from build123d import *

# Parameters (mm, degrees)
SKETCH1_W           = 288
SKETCH1_H           = 50
BOSS_EXTRUDE1_DEPTH = 5
SKETCH2_R           = 1.5
CUT_EXTRUDE1_DEPTH  = 5
SKETCH3_W           = 30
SKETCH3_H           = 45
BOSS_EXTRUDE2_DEPTH = 5
FILLET1_R           = 10
SKETCH4_W           = 5
SKETCH4_H           = 5
CUT_EXTRUDE2_DEPTH  = 5
SKETCH5_R           = 1.7
CUT_EXTRUDE3_DEPTH  = 5
SKETCH7_R           = 2
CUT_EXTRUDE4_DEPTH  = 10


with BuildPart() as part:
    # Sketch1 → Boss-Extrude1 (new body)
    with BuildSketch(Plane(origin=(0, 0, 0), x_dir=(1, 0, 0), z_dir=(0, 1, 0))):
        Rectangle(SKETCH1_W, SKETCH1_H)
    extrude(amount=BOSS_EXTRUDE1_DEPTH)

    # Sketch2 → Cut-Extrude1 (cut)
    with BuildSketch(Plane(origin=(0, 5, 0), x_dir=(1, 0, 0), z_dir=(0, 1, 0))):
        with Locations((-130, 10)):
            Circle(SKETCH2_R)
        with Locations((-110, 10)):
            Circle(SKETCH2_R)
        with Locations((-110, -10)):
            Circle(SKETCH2_R)
        with Locations((-130, -10)):
            Circle(SKETCH2_R)
        with Locations((130, -10)):
            Circle(SKETCH2_R)
        with Locations((110, -10)):
            Circle(SKETCH2_R)
        with Locations((110, 10)):
            Circle(SKETCH2_R)
        with Locations((130, 10)):
            Circle(SKETCH2_R)
    extrude(amount=-CUT_EXTRUDE1_DEPTH, mode=Mode.SUBTRACT)

    # Sketch3 → Boss-Extrude2 (add)
    with BuildSketch(Plane(origin=(0, 5, 0), x_dir=(1, 0, 0), z_dir=(0, 1, 0))):
        with Locations((-129, 47.5)):
            Rectangle(SKETCH3_W, SKETCH3_H)
        with Locations((-129, -47.5)):
            Rectangle(SKETCH3_W, SKETCH3_H)
        with Locations((129, -47.5)):
            Rectangle(SKETCH3_W, SKETCH3_H)
        with Locations((129, 47.5)):
            Rectangle(SKETCH3_W, SKETCH3_H)
    extrude(amount=-BOSS_EXTRUDE2_DEPTH)

    # Fillet1
    fillet1_edges = [part.edges().sort_by_distance(p)[0] for p in [
        (-114, 2.5, -25),
        (-114, 2.5, 25),
        (114, 2.5, 25),
        (114, 2.5, -25),
    ]]
    fillet(fillet1_edges, radius=FILLET1_R)

    # Sketch4 → Cut-Extrude2 (cut)
    with BuildSketch(Plane(origin=(0, 5, 0), x_dir=(1, 0, 0), z_dir=(0, 1, 0))):
        with Locations((10, 10)):
            Rectangle(SKETCH4_W, SKETCH4_H)
        with Locations((-10, 10)):
            Rectangle(SKETCH4_W, SKETCH4_H)
        with Locations((-10, -10)):
            Rectangle(SKETCH4_W, SKETCH4_H)
        with Locations((10, -10)):
            Rectangle(SKETCH4_W, SKETCH4_H)
    extrude(amount=-CUT_EXTRUDE2_DEPTH, mode=Mode.SUBTRACT)

    # Sketch5 → Cut-Extrude3 (cut)
    with BuildSketch(Plane(origin=(0, 5, 0), x_dir=(1, 0, 0), z_dir=(0, 1, 0))):
        with Locations((0, 10)):
            Circle(SKETCH5_R)
        with Locations((0, -10)):
            Circle(SKETCH5_R)
        with Locations((10, 0)):
            Circle(SKETCH5_R)
        with Locations((-10, 0)):
            Circle(SKETCH5_R)
    extrude(amount=-CUT_EXTRUDE3_DEPTH, mode=Mode.SUBTRACT)

    # Sketch7 → Cut-Extrude4 (cut)
    with BuildSketch(Plane(origin=(0, 5, 0), x_dir=(1, 0, 0), z_dir=(0, 1, 0))):
        with Locations((-136.5, 45)):
            Circle(SKETCH7_R)
        with Locations((-136.5, -30)):
            Circle(SKETCH7_R)
        with Locations((136.5, -30)):
            Circle(SKETCH7_R)
        with Locations((136.5, 45)):
            Circle(SKETCH7_R)
    extrude(amount=-CUT_EXTRUDE4_DEPTH, mode=Mode.SUBTRACT)


solid = part.part
Geometry: final body of the model. Coordinates: model frame, mm. A direction names the side the tool comes from. Give positions to 0.01 mm unless a question says otherwise; leave off trailing zeros. Loops run counter-clockwise (first coordinate to the right, second up) from the corner with the lowest first, then second, coordinate; pieces in that order, holes last. Notation, with made-up numbers: M 16.25,62.5 L 74.25,62.5 A27 cw 74.25,89.5 Z; hole C 69,50.25 d3. An arc over 180 degrees is marked long. Put each result on its own line as item: value.
1) Cut plane C-C, the plane x = 73. Return the cut outline in (y, z), plus the area to 3 significant figures.
Computed values:
outline: M 0,-25 L 5,-25 L 5,25 L 0,25 Z
area: 250 mm^2
2) Cut plane B-B, the plane y = 4.1. Give the number of separate pieces and of enclosed holes in the cut face, plus the area to 3 significant figures.
Computed values:
separate pieces: 1
enclosed holes: 20
area: 19,600 mm^2
3) Mould query, pull axis X, two halves, no side actions, for faces 5 (the flat face through (10, 3, 12.5)), 6 (the flat face through (-10, 3, 7.5)), 7 (the flat face through (-144, 3, 1)), 8 (the flat face through (129, 3, -70)). Classes: released by +X, released by -X, zero draft, split by the parting line, or undercut.
Computed values:
face 5: undercut
face 6: undercut
face 7: released by -X
face 8: zero draft
4) Cut plane A-A, the plane z = 58. Return the cut outline in (x, y), plus the area to 3 significant figures.
Computed values:
outline: M -144,0 L -114,0 L -114,5 L -144,5 Z; M 114,0 L 144,0 L 144,5 L 114,5 Z
area: 300 mm^2
5) Material intervals for L1, parallel to Z at x = -136.5, y = 2.85; L2, parallel to Z at x = 0, y = 2.45; L3, parallel to Z at x = 10, y = 1.6, sorted ascending. Write a range as from..to.
Computed values:
L1: z = -70..-47, -43..28, 32..70
L2: z = -25..-11.7, -8.3..8.3, 11.7..25
L3: z = -25..-12.5, -7.5..-1.7, 1.7..7.5, 12.5..25
6) Reachability of faces 1 (the cylindrical face through (111.15, 2.46, 28.01)), 2 (the flat face through (-12.5, 3, 10)), 3 (the cylindrical face through (-111.15, 2.46, -28.01)), 4 (the flat face through (-2, 5, -1)) from +Z, -Z, +X, -X, +Y, -Y: full face, straight path, thin tool, end or side. Return the list, or none.
Computed values:
face 1: +Z, +Y, -Y
face 2: +Y, -Y
face 3: -Z, +Y, -Y
face 4: +Z, -Z, +X, -X, +Y
7) First-contact query: P1, Ø5, axis at x = -110, z = -10, coming from the -Y side; P2, Ø1.5, axis at x = -9.5, y = 1.5, coming from the -Z side; P3, Ø2.5, axis at x = -10.5, y = 3.5, coming from the +Z side. Flat tips, straight axial feed; report the tip coordinate or a pass-through.
Computed values:
P1: stops at y = 0
P2: stops at z = -25
P3: stops at z = 25
